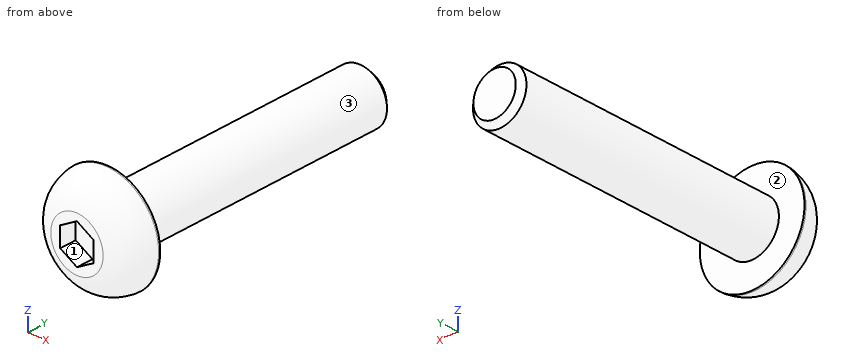
from build123d import *

# Parameters (mm, degrees)
SKETCH1_R           = 4.7
BOSS_EXTRUDE1_DEPTH = 3
SKETCH2_R           = 2.4
BOSS_EXTRUDE2_DEPTH = 25
CUT_EXTRUDE1_DEPTH  = 1.5
CHAMFER1_SIZE       = 0.5


with BuildPart() as part:
    # Sketch1 → Boss-Extrude1 (new body)
    with BuildSketch(Plane(origin=(0, 0, 0), x_dir=(1, 0, 0), z_dir=(0, 1, 0))):
        Circle(SKETCH1_R)
    extrude(amount=BOSS_EXTRUDE1_DEPTH)

    # Sketch2 → Boss-Extrude2 (add)
    with BuildSketch(Plane(origin=(0, 3, 0), x_dir=(1, 0, 0), z_dir=(0, 1, 0))):
        Circle(SKETCH2_R)
    extrude(amount=BOSS_EXTRUDE2_DEPTH)

    # Sketch3 → Cut-Revolve1 (revolve, cut)
    with BuildSketch(Plane.XY):
        with BuildLine():
            Line((2.35, 0), (4.7, 0))
            Line((4.7, 0), (4.7, 2.85))
            add(Edge.make_bspline(
                [(2.35, 0), (4.432462228, 0.599611143), (4.7, 2.85)],
                knots=[0, 0, 0, 1, 1, 1], degree=2))
        make_face()
    revolve(axis=Axis((0, 0, 0), (0, 1, 0)), mode=Mode.SUBTRACT)

    # Sketch4 → Cut-Extrude1 (cut)
    with BuildSketch(Plane.XZ):
        Polygon((0, 1.732050808), (-1.5, 0.866025404), (-1.5, -0.866025404), (0, -1.732050808), (1.5, -0.866025404), (1.5, 0.866025404), align=None)
    extrude(amount=-CUT_EXTRUDE1_DEPTH, mode=Mode.SUBTRACT)

    # Chamfer1
    chamfer1_edges = [part.edges().sort_by_distance(p)[0] for p in [
        (-2.4, 28, 0),
    ]]
    chamfer(chamfer1_edges, length=CHAMFER1_SIZE)


solid = part.part
For this review, take the finished solid that the model builds, in its own axes (mm). Face numbers are marked on the shaded views. Round coordinates to 2 decimals unless told otherwise and drop trailing zeros. Order: outer loops, then holes, each group sorted by start corner. A loop starts at its lowest first (then second) coordinate and runs counter-clockwise, first axis right, second up. Notation, with made-up numbers: M -22,-16 L 13,-16 A15 ccw 13,5 Z; hole C -27.75,9.5 d1. An arc over 180 degrees is marked long. Use a Markdown table: item, result. Add a question column.
Item 1: Insertion check: pin 1 (3 mm diameter, centred on x = -2, y = 3, fed in from -Z); pin 2 (1.5 mm diameter, centred on x = 3, z = 0, fed in from +Y); pin 3 (0.8 mm diameter, centred on y = 0.5, z = 0, fed in from -X). Each pin has a flat end and moves straight along its axis. Give the tip position at first contact, or say it passes through.
Item 2: Mouldability with a two-part tool opening along X and no side actions: class the marked faces 1, 2 and 3 as released by +X, released by -X, zero draft, split by the parting line, or undercut.
Item 3: To check wall thickness, follow line 1 along X through (y, z) = (3.5, 0); line 2 along Z through (x, y) = (-0.5, 11.25); line 3 along Y through (x, z) = (-0.75, 1.75). State the ranges of each line that lie inside material, in increasing order.
Item 4: Add section A-A, the plane y = 6.75. Give the boundary of the cut face in (x, z), then the cut area to 3 significant figures.
Geometry results:
| question | item | result |
|---|---|---|
| 1 | pin 1 | stops at z = -4.67 |
| 1 | pin 2 | stops at y = 27.65 |
| 1 | pin 3 | stops at x = -3.88 |
| 2 | face 1 | undercut |
| 2 | face 2 | zero draft |
| 2 | face 3 | split by the parting line |
| 3 | line 1 | x = -2.4 to 2.4 |
| 3 | line 2 | z = -2.35 to 2.35 |
| 3 | line 3 | y = 0 to 28 |
| 4 | outline | C 0,0 d4.8 |
| 4 | area | 18.1 mm² |
